For this review, use the dimensioned drawing (mm, ordinates from the lowest corner) and the shaded views. A direction names the side the tool comes from. Coordinates: 2 decimals unless noted, no trailing zeros. Loops run counter-clockwise (first coordinate to the right, second up) from the corner with the lowest first, then second, coordinate; pieces in that order, holes last. Notation, with made-up numbers: (-4.75, 61.5) -> (50.25, 61.5) arc R34 cw to (50.25, 98.5) -> close; hole circle Ø5 at (15, -1). An arc over 180 degrees is marked (long way). One line per question, with ' | ' between items. Start each with the question number.
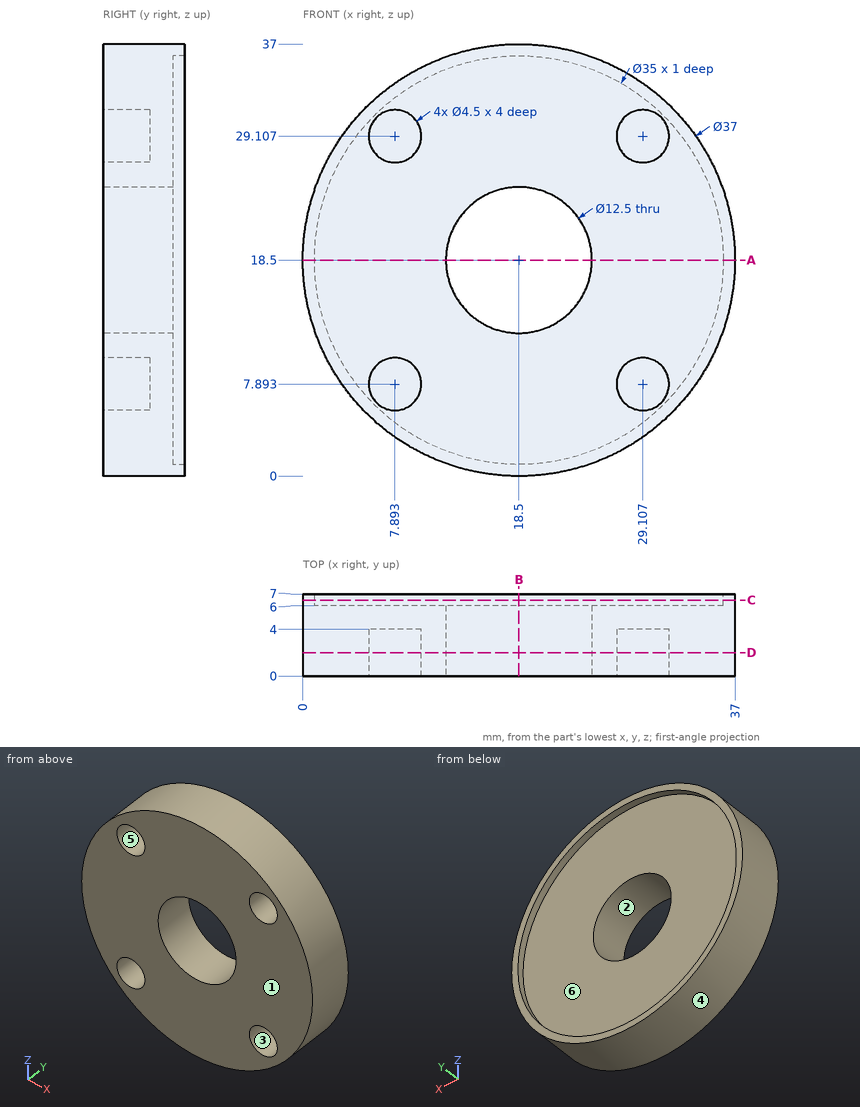
1) Consider section D-D, the plane y = 2. Write out the cut boundary in (x, z), plus the area to 3 significant figures.
2) Consider section C-C, the plane y = 6.5. Write out the cut boundary in (x, z).
3) Machinability: for the marked faces 5 and 6, which of the approach directions +Z, -Z, +X, -X, +Y, -Y give a long, thin tool a straight path to every point of the face, cutting with its end or side? Answer none if there is none.
4) Consider section A-A, the plane z = 18.5. Write out the cut boundary in (x, y).
5) Mouldability with a two-part tool opening along Z and no side actions: class the marked faces 1, 2, 3 and 4 as +Z half, -Z half, draft (parallel to the pull), parting line (faces both ways), or undercut.
6) Wall thickness on L1, parallel to X at y = 2, z = 9.5 (1 decimal); L2, parallel to X at y = 6.5, z = 18.5; L3, parallel to Z at x = 18.5, y = 4.55: over which ranges is each line inside the solid? List them lowest first.
7) Insertion check: pin 1 Ø2.5 at (x, z) = (7.89, 7.89) entering from -Y; pin 2 Ø4 at (x, z) = (7.89, 29.11) entering from +Y; pin 3 Ø3.5 at (x, z) = (8.5, 29.5) entering from -Y; pin 4 Ø1 at (y, z) = (2.5, 13.5) entering from +X (1 decimal). Each pin has a flat end and moves straight along its axis. Give the tip position at first contact, or say it passes through.
8) Consider section B-B, the plane x = 18.5. Write out the cut boundary in (y, z).
Filled sheet:
1) outline: circle Ø37 at (18.5, 18.5); hole circle Ø4.5 at (7.89, 7.89); hole circle Ø4.5 at (7.89, 29.11); hole circle Ø12.5 at (18.5, 18.5); hole circle Ø4.5 at (29.11, 7.89); hole circle Ø4.5 at (29.11, 29.11) | area: 889 mm^2
2) outline: circle Ø37 at (18.5, 18.5); hole circle Ø35 at (18.5, 18.5)
3) face 5: -Y | face 6: +Y
4) outline: (0, 0) -> (12.25, 0) -> (12.25, 6) -> (1, 6) -> (1, 7) -> (0, 7) -> close; (24.75, 0) -> (37, 0) -> (37, 7) -> (36, 7) -> (36, 6) -> (24.75, 6) -> close
5) face 1: draft | face 2: undercut | face 3: undercut | face 4: parting line
6) L1: 2.3 to 6.3, 9.5 to 27.5, 30.7 to 34.7 | L2: 0 to 1, 36 to 37 | L3: 0 to 12.25, 24.75 to 37
7) pin 1: y = 4 | pin 2: y = 6 | pin 3: y = 0 | pin 4: x = 36.4
8) outline: (0, 0) -> (7, 0) -> (7, 1) -> (6, 1) -> (6, 12.25) -> (0, 12.25) -> close; (0, 24.75) -> (6, 24.75) -> (6, 36) -> (7, 36) -> (7, 37) -> (0, 37) -> close
